The listing builds one solid part. Answer for the finished solid, in the listing's coordinates (mm). A direction names the side the tool comes from. Give positions to 0.01 mm unless a question says otherwise; leave off trailing zeros. Order: outer loops, then holes, each group sorted by start corner. A loop starts at its lowest first (then second) coordinate and runs counter-clockwise, first axis right, second up. Notation, with made-up numbers: (-32.75, 36.25) - (-26.75, 36.25) arc R14 ccw to (-26.75, 41.25) - close; hole circle Ø10 at (79, 18). An arc over 180 degrees is marked (long way). Use CSV: the item, a comma, the result in double quotes.
```python
from build123d import *

# Parameters (mm, degrees)
SKETCH1_W           = 3
SKETCH1_H           = 12
BOSS_EXTRUDE1_DEPTH = 5
FILLET3_R           = 20
FILLET4_R           = 20
FILLET5_R           = 20


with BuildPart() as part:
    # Sketch1 → Boss-Extrude1 (new body)
    # profile 1 of 4: a face of its own
    with BuildSketch(Plane(origin=(0, 0, 0), x_dir=(1, 0, 0), z_dir=(0, 1, 0))):
        with BuildLine():
            Line((0, 0), (75, 0))
            Line((75, 0), (75, 76))
            Line((75, 76), (58.25, 76))
            ThreePointArc((58.25, 76), (55.689339828, 74.939339828), (56.75, 77.5))
            Line((56.75, 77.5), (56.75, 110.5))
            ThreePointArc((56.75, 110.5), (55.689339828, 113.060660172), (58.25, 112))
            Line((58.25, 112), (75, 112))
            Line((75, 112), (75, 183.494931242))
            ThreePointArc((75, 183.494931242), (64.75, 193.744931242), (75, 203.994931242))
            Line((75, 203.994931242), (75, 223))
            Line((75, 223), (25, 223))
            Line((25, 223), (0, 223))
            Line((0, 223), (0, 187))
            Line((0, 187), (25, 187))
            Line((25, 187), (25, 132.991356344))
            Line((25, 132.991356344), (28, 132.991356344))
            Line((28, 132.991356344), (28, 120.991356344))
            Line((28, 120.991356344), (25, 120.991356344))
            Line((25, 120.991356344), (25, 112))
            Line((25, 112), (0, 111.5))
            Line((0, 111.5), (0, 0))
        make_face()
        with Locations((45, 126.991356344)):
            Rectangle(SKETCH1_W, SKETCH1_H, mode=Mode.SUBTRACT)
    # profile 2 of 4: a face of its own
    with BuildSketch(Plane(origin=(0, 0, 0), x_dir=(1, 0, 0), z_dir=(0, 1, 0))):
        with BuildLine():
            Line((75, 76), (75, 0))
            Line((75, 0), (150, 0))
            Line((150, 0), (150, 111.5))
            Line((150, 111.5), (125, 112))
            Line((125, 112), (125, 120.991356344))
            Line((125, 120.991356344), (122, 120.991356344))
            Line((122, 120.991356344), (122, 132.991356344))
            Line((122, 132.991356344), (125, 132.991356344))
            Line((125, 132.991356344), (125, 187))
            Line((125, 187), (150, 187))
            Line((150, 187), (150, 223))
            Line((150, 223), (75, 223))
            Line((75, 223), (75, 203.994931242))
            ThreePointArc((75, 203.994931242), (82.247844507, 200.992775749), (85.25, 193.744931242))
            ThreePointArc((85.25, 193.744931242), (82.247844507, 186.497086735), (75, 183.494931242))
            Line((75, 183.494931242), (75, 112))
            Line((75, 112), (91.75, 112))
            ThreePointArc((91.75, 112), (93.25, 113.5), (94.75, 112))
            ThreePointArc((94.75, 112), (94.310660172, 110.939339828), (93.25, 110.5))
            Line((93.25, 110.5), (93.25, 77.5))
            ThreePointArc((93.25, 77.5), (94.310660172, 77.060660172), (94.75, 76))
            ThreePointArc((94.75, 76), (93.25, 74.5), (91.75, 76))
            Line((91.75, 76), (75, 76))
        make_face()
        with Locations((105, 126.991356344)):
            Rectangle(SKETCH1_W, SKETCH1_H, mode=Mode.SUBTRACT)
    # profile 3 of 4: a face of its own
    with BuildSketch(Plane(origin=(0, 0, 0), x_dir=(1, 0, 0), z_dir=(0, 1, 0))):
        with BuildLine():
            Line((75, 112), (75, 76))
            Line((75, 76), (91.75, 76))
            ThreePointArc((91.75, 76), (92.189339828, 77.060660172), (93.25, 77.5))
            Line((93.25, 77.5), (93.25, 110.5))
            ThreePointArc((93.25, 110.5), (92.189339828, 110.939339828), (91.75, 112))
            Line((91.75, 112), (75, 112))
        make_face()
    # profile 4 of 4: a face of its own
    with BuildSketch(Plane(origin=(0, 0, 0), x_dir=(1, 0, 0), z_dir=(0, 1, 0))):
        with BuildLine():
            Line((58.25, 76), (75, 76))
            Line((75, 76), (75, 112))
            Line((75, 112), (58.25, 112))
            ThreePointArc((58.25, 112), (57.810660172, 110.939339828), (56.75, 110.5))
            Line((56.75, 110.5), (56.75, 77.5))
            ThreePointArc((56.75, 77.5), (57.810660172, 77.060660172), (58.25, 76))
        make_face()
    extrude(amount=BOSS_EXTRUDE1_DEPTH)

    # Fillet3
    fillet3_edges = [part.edges().sort_by_distance(p)[0] for p in [
        (0, 2.5, -223),
    ]]
    fillet(fillet3_edges, radius=FILLET3_R)

    # Fillet4
    fillet4_edges = [part.edges().sort_by_distance(p)[0] for p in [
        (150, 2.5, -223),
    ]]
    fillet(fillet4_edges, radius=FILLET4_R)

    # Fillet5
    fillet5_edges = [part.edges().sort_by_distance(p)[0] for p in [
        (150, 2.5, -111.5),
        (150, 2.5, 0),
        (0, 2.5, 0),
        (0, 2.5, -111.5),
    ]]
    fillet(fillet5_edges, radius=FILLET5_R)


solid = part.part
```
Item 1: Which of the six approach directions +Z, -Z, +X, -X, +Y, -Y give full straight-line access (tool end or side, diameter ignored) to faces 1 (the face through (0, 2, -195)), 2 (the face through (43.5, 2, -127)), 3 (the face through (144.13, 2.54, -106.05)), 4 (the face through (5.87, 2.54, -106.05))?
Taken from the geometry:
face 1,"+Z, -Z, -X, +Y, -Y"
face 2,"+Y, -Y"
face 3,"+X, +Y, -Y"
face 4,"-X, +Y, -Y"
Item 2: The part is cut by section A-A (x = 14.5). Give the vertices of the cut face in (y, z).
Taken from the geometry:
outline,"(0, -222.23) - (5, -222.23) - (5, -187) - (0, -187) - close; (0, -111.12) - (5, -111.12) - (5, -0.77) - (0, -0.77) - close"
Item 3: The part is cut by section D-D (x = 139). Give the vertices of the cut face in (y, z), and give its area (3 significant figures).
Taken from the geometry:
outline,"(0, -220.86) - (5, -220.86) - (5, -187) - (0, -187) - close; (0, -109.76) - (5, -109.76) - (5, -2.14) - (0, -2.14) - close"
area,"707 mm^2"
Item 4: Find the intervals of material crossed by line 1 along X through (y, z) = (2.35, -76); line 2 along Z through (x, y) = (56.75, 3.7); line 3 along X through (y, z) = (0.35, -123.5), in increasing order.
Taken from the geometry:
line 1,"0 to 55.25, 58.25 to 91.75, 94.75 to 150"
line 2,"-223 to -113.5, -110.5 to -77.5, -74.5 to 0"
line 3,"28 to 43.5, 46.5 to 103.5, 106.5 to 122"
Item 5: The part is cut by section C-C (z = -141). Give the vertices of the cut face in (x, y), and give its area (3 significant figures).
Taken from the geometry:
outline,"(25, 0) - (125, 0) - (125, 5) - (25, 5) - close"
area,"500 mm^2"
Item 6: The mould has two halves that part along Z. Classify faces 5 (the face through (74, 0, -113)), 6 (the face through (5.703, 2.535, -216.986)), 7 (the face through (12, 2, -187)): +Z half, -Z half, draft (parallel to the pull), parting line (faces both ways), or undercut.
Taken from the geometry:
face 5,"draft"
face 6,"-Z half"
face 7,"undercut"
Item 7: Each of these flat-tipped pins is pushed along its axis until it touches: pin 1 (1.5 mm diameter, centred on y = 4, z = -123, fed in from +X); pin 2 (2.5 mm diameter, centred on x = 56.75, z = -112, fed in from -Y); pin 3 (2 mm diameter, centred on y = 2, z = -109, fed in from +X); pin 4 (10 mm diameter, centred on x = 48, z = -186, fed in from -Y). Where does it stop, or does it pass through?
Taken from the geometry:
pin 1,"x = 122"
pin 2,"through"
pin 3,"x = 141.86"
pin 4,"y = 0"
Item 8: The part is cut by section B-B (y = 4.2). Count the separate pieces of the cut face and the enclosed holes in it, and give its area (3 significant figures).
Taken from the geometry:
separate pieces,"1"
enclosed holes,"7"
area,"28,700 mm^2"
